Design review of the part shown in the three views and the two pictorial views. Dimensions are in mm from the part's minimum x, y and z. Round coordinates to 2 decimals unless told otherwise and drop trailing zeros. Order: outer loops, then holes, each group sorted by start corner. A loop starts at its lowest first (then second) coordinate and runs counter-clockwise, first axis right, second up. Notation, with made-up numbers: M 85.5,-31 L 141.5,-31 A19 ccw 141.5,-25 Z; hole C -22,29.25 d3. An arc over 180 degrees is marked long. Write each question's results on one line, items separated by ' | '. Start each with the question number.
Item 1: Wall thickness on line 1 (X direction, y = 2.15, z = 29); line 2 (Z direction, x = 28.5, y = 2.75); line 3 (Y direction, x = 43, z = 12.5): over which ranges is each line inside the solid? List them lowest first. Write a range as [from, to].
Item 2: Clearance check with flat-ended pins moving along their axes: pin 1 (8 mm diameter, centred on x = 8, z = 10, fed in from +Y); pin 2 (1.5 mm diameter, centred on x = 9, y = 2.5, fed in from -Z); pin 3 (4 mm diameter, centred on x = 35.5, y = 4.5, fed in from +Z); pin 4 (6 mm diameter, centred on x = 29, z = 5, fed in from -Y). State where each tip first meets the part, or that it passes through.
Item 3: The part is to be moulded in two halves that separate along X. For the marked faces 1, 2 and 3, say which applies: +X half, -X half, draft (parallel to the pull), parting line (faces both ways), or undercut.
Item 4: Take a section at A-A, the plane z = 29. Write out the cut boundary in (x, y).
Item 5: Take a section at D-D, the plane x = 5. Write out the cut boundary in (y, z).
Item 6: Take a section at B-B, the plane x = 29. Write out the cut boundary in (y, z), plus the area to 4 significant figures.
Item 7: Take a section at C-C, the plane z = 53. Write out the cut boundary in (x, y), plus the area to 3 significant figures.
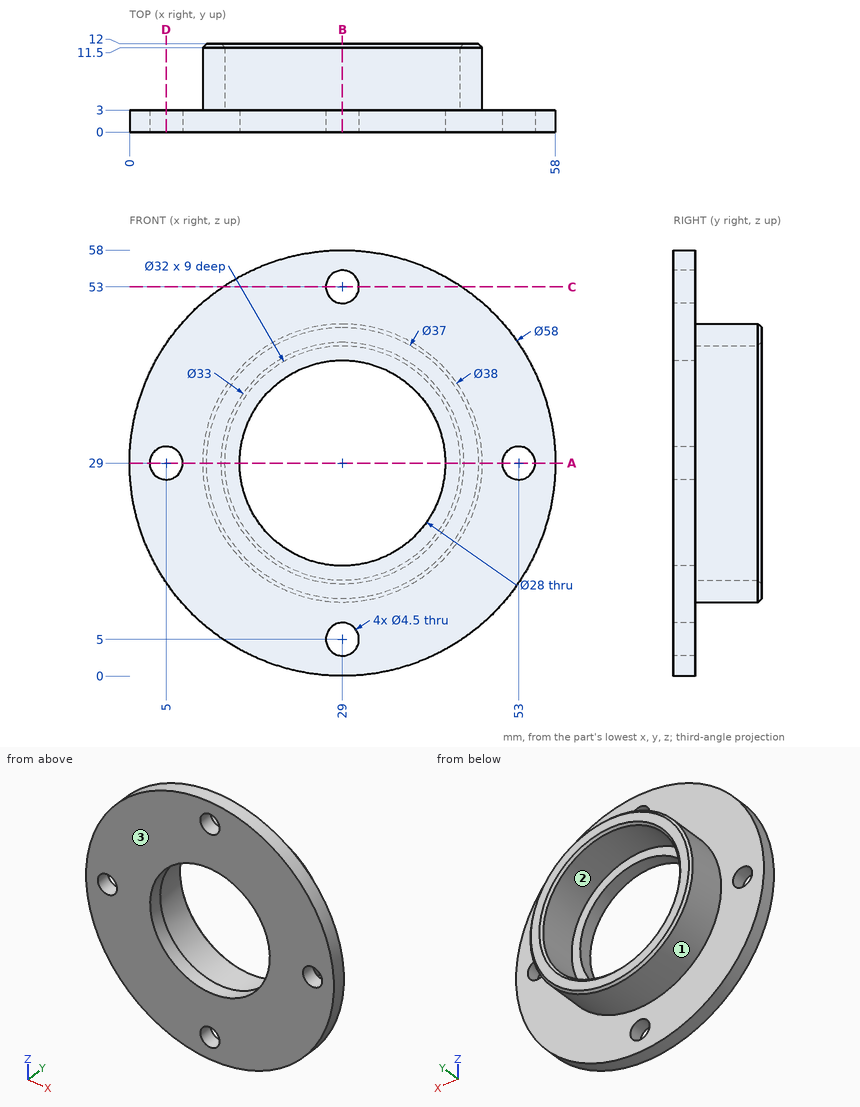
Results list:
1) line 1: [0, 2.75], [7.25, 15], [43, 50.75], [55.25, 58] | line 2: [0, 2.81], [7.19, 15.01], [42.99, 50.81], [55.19, 58] | line 3: [0, 3]
2) pin 1: y = 3 | pin 2: z = 7.31 | pin 3: z = 57.53 | pin 4: y = 0
3) face 1: parting line | face 2: undercut | face 3: draft
4) outline: M 0,0 L 2.75,0 L 2.75,3 L 0,3 Z; M 7.25,0 L 15,0 L 15,3 L 13,3 L 13,11.5 L 12.5,12 L 10.5,12 L 10,11.5 L 10,3 L 7.25,3 Z; M 43,0 L 50.75,0 L 50.75,3 L 48,3 L 48,11.5 L 47.5,12 L 45.5,12 L 45,11.5 L 45,3 L 43,3 Z; M 55.25,0 L 58,0 L 58,3 L 55.25,3 Z
5) outline: M 0,12.72 L 3,12.72 L 3,26.75 L 0,26.75 Z; M 0,31.25 L 3,31.25 L 3,45.28 L 0,45.28 Z
6) outline: M 0,0 L 3,0 L 3,2.75 L 0,2.75 Z; M 0,7.25 L 3,7.25 L 3,10 L 11.5,10 L 12,10.5 L 12,12.5 L 11.5,13 L 3,13 L 3,15 L 0,15 Z; M 0,43 L 3,43 L 3,45 L 11.5,45 L 12,45.5 L 12,47.5 L 11.5,48 L 3,48 L 3,50.75 L 0,50.75 Z; M 0,55.25 L 3,55.25 L 3,58 L 0,58 Z | area: 116.5 mm²
7) outline: M 12.72,0 L 26.75,0 L 26.75,3 L 12.72,3 Z; M 31.25,0 L 45.28,0 L 45.28,3 L 31.25,3 Z | area: 84.2 mm²
